CAD build for the part. Positions are in the model's coordinates, mm. A direction names the side the tool comes from. Coordinates: 2 decimals unless noted, no trailing zeros. Order: outer loops, then holes, each group sorted by start corner. A loop starts at its lowest first (then second) coordinate and runs counter-clockwise, first axis right, second up. Notation, with made-up numbers: (-23, -14.75) - (7, -14.75) arc R21 ccw to (7, -6.75) - close; hole circle Ø5 at (32, 23.5). An arc over 180 degrees is marked (long way). Use one line per item in the form item = value.
Autodesk Inventor part; units mm, degrees
ref_plane "YZ Plane" through (0, 0, 0) normal (1, 0, 0) x (0, 1, 0)
ref_plane "XZ Plane" through (0, 0, 0) normal (0, 1, 0) x (-1, 0, 0)
ref_plane "XY Plane" through (0, 0, 0) normal (0, 0, 1) x (1, 0, 0)
sketch "Sketch1" plane through (0, 0, 0) normal (0, 0, 1) x (1, 0, 0)
  line L0 (-5.7995, -0.4901) -> (0.2005, -0.4901)
  line L1 (0.2005, -0.4901) -> (0.2005, 2.5099)
  line L2 (0.2005, 2.5099) -> (10.2005, 2.5099)
  line L3 (10.2005, 2.5099) -> (10.2005, -0.4901)
  line L4 (10.2005, -0.4901) -> (16.2005, -0.4901)
  line L5 (16.2005, -0.4901) -> (16.2005, 1.5099)
  line L6 (16.2005, 1.5099) -> (12.2005, 1.5099)
  line L7 (12.2005, 1.5099) -> (12.2005, 4.5099)
  line L8 (12.2005, 4.5099) -> (-1.7995, 4.5099)
  line L9 (-1.7995, 4.5099) -> (-1.7995, 1.5099)
  line L10 (-1.7995, 1.5099) -> (-5.7995, 1.5099)
  line L11 (-5.7995, 1.5099) -> (-5.7995, -0.4901)
  point P0 (0, 0)
  dimension "d0" = 3
  dimension "d1" = 2
  dimension "d2" = 2
  dimension "d3" = 2
  dimension "d4" = 2
  dimension "d5" = 2
  dimension "d6" = 10
  dimension "d7" = 6
  dimension "d8" = 6
extrude "Extrusion1" add sketch "Sketch1" along normal blind 8
sketch "Sketch2" plane through (12.2005, 1.5099, 0) normal (0, 1, 0) x (1, 0, 0)
  line L0 (-14, 0) -> (-18, 0)
  line L1 (-18, 0) -> (-18, -8)
  line L2 (-14, -8) -> (-18, -8)
  line L3 (-14, 0) -> (-14, -8)
  line L4 (4, 0) -> (0, 0)
  line L5 (0, 0) -> (0, -8)
  line L6 (4, -8) -> (0, -8)
  line L7 (4, 0) -> (4, -8)
  point P0 (-12.2005, 0)
  point P1 (-16, -1.8)
  point P2 (-16, -6.2)
  point P3 (2, -1.8)
  point P4 (2, -6.2)
  dimension "d11" = 1.8
  dimension "d12" = 1.8
  dimension "d13" = 2
  dimension "d14" = 2
hole "Hole1" at (-3.7995, 1.5099, 1.8) at (-3.7995, 1.5099, 6.2) at (14.2005, 1.5099, 1.8) at (14.2005, 1.5099, 6.2) direction (0, -1, 0) diameter 1.6 depth 8 tip angle 118
fillet "Fillet1" radius 1.5 4 edges at (16.2005, 0.5099, 0) (16.2005, 0.5099, 8) (-5.7995, 0.5099, 0) (-5.7995, 0.5099, 8)
fillet "Fillet2" radius 0.25 4 edges at (12.2005, 4.5099, 4) (12.2005, 1.5099, 4) (-1.7995, 1.5099, 4) (-1.7995, 4.5099, 4)
chamfer "Chamfer1" distance 0.8 distance2 2 1 edges at (5.2005, 2.5099, 8) measured on face at (3.5338, 3.8432, 8)
chamfer "Chamfer2" distance 0.8 distance2 2 1 edges at (0.2005, 1.0099, 8) measured on face at (3.5338, 4.1099, 8)
chamfer "Chamfer3" distance 0.8 distance2 2 1 edges at (10.2005, 1.0099, 8) measured on face at (3.5338, 4.1099, 8)
equation "\"d2\" = d1"
equation "\"d3\" = d1"
equation "\"d4\" = d1"
equation "\"d5\" = d1"
equation "\"d7\" = d8"
properties part number "CNCM_ALU_Visial_inspection_tray_bucket_mount" material "Aluminum 6061"
Item 1: Cut at C-C, the plane x = -4. Write the cut outline in (y, z).
Derived:
outline = (-0.49, 0) - (1.51, 0) - (1.51, 1.03) - (-0.49, 1.03) - close; (-0.49, 2.57) - (1.51, 2.57) - (1.51, 5.43) - (-0.49, 5.43) - close; (-0.49, 6.97) - (1.51, 6.97) - (1.51, 8) - (-0.49, 8) - close
Item 2: Drop flat-ended pins along their axis: pin 1 (2 mm diameter, centred on y = 3, z = 7, fed in from -X); pin 2 (3 mm diameter, centred on x = 6.5, z = 4, fed in from -Y); pin 3 (0.8 mm diameter, centred on y = 3.5, z = 5.5, fed in from +X); pin 4 (1.4 mm diameter, centred on x = -3.8, z = 1.8, fed in from -Y). Give the stop position or say it passes through.
Derived:
pin_1 = -1.8
pin_2 = 2.51
pin_3 = 12.2
pin_4 = through
Item 3: Two-plate mould, pull along X, no slides. Class faces 1 (the face through (10.6, 1.4, 7)), 2 (the face through (-5.37, 0.5, 0.45)), 3 (the face through (5, 4.51, 4)): +X half, -X half, draft (parallel to the pull), parting line (faces both ways), or undercut.
Derived:
face_1 = undercut
face_2 = -X half
face_3 = draft
Item 4: Cut at D-D, the plane z = 4. Write the cut outline in (x, y).
Derived:
outline = (-5.8, -0.49) - (0.2, -0.49) - (0.2, 2.51) - (10.2, 2.51) - (10.2, -0.49) - (16.2, -0.49) - (16.2, 1.51) - (12.45, 1.51) arc R0.25 cw to (12.2, 1.76) - (12.2, 4.26) arc R0.25 ccw to (11.95, 4.51) - (-1.55, 4.51) arc R0.25 ccw to (-1.8, 4.26) - (-1.8, 1.76) arc R0.25 cw to (-2.05, 1.51) - (-5.8, 1.51) - close
Item 5: Drill centre lines: line 1 (X direction, y = 0.9, z = 1.8); line 2 (X direction, y = 0.3, z = 4.5); line 3 (X direction, y = 1, z = 6.2). Where is each one in solid material? Low to high. Write a range as [from, to].
Derived:
line_1 = [-5.8, -4.6], [-3, 0.2], [10.2, 13.4], [15, 16.2]
line_2 = [-5.8, 0.2], [10.2, 16.2]
line_3 = [-5.8, -4.6], [-3, 0.12], [10.28, 13.4], [15, 16.2]
Item 6: Cut at B-B, the plane y = 0.6. Write the cut outline in (x, z).
Derived:
outline = (-5.8, 1.5) arc R1.5 ccw to (-4.3, 0) - (0.2, 0) - (0.2, 6) - (-0.6, 8) - (-4.3, 8) arc R1.5 ccw to (-5.8, 6.5) - close; (10.2, 0) - (14.7, 0) arc R1.5 ccw to (16.2, 1.5) - (16.2, 6.5) arc R1.5 ccw to (14.7, 8) - (11, 8) - (10.2, 6) - close; hole circle Ø1.6 at (-3.8, 1.8); hole circle Ø1.6 at (-3.8, 6.2); hole circle Ø1.6 at (14.2, 1.8); hole circle Ø1.6 at (14.2, 6.2)
Item 7: Cut at A-A, the plane z = 1.8. Write the cut outline in (x, y), plus the area to 3 significant figures.
Derived:
outline = (-5.8, -0.49) - (-4.6, -0.49) - (-4.6, 1.51) - (-5.8, 1.51) - close; (-3, -0.49) - (0.2, -0.49) - (0.2, 2.51) - (10.2, 2.51) - (10.2, -0.49) - (13.4, -0.49) - (13.4, 1.51) - (12.45, 1.51) arc R0.25 cw to (12.2, 1.76) - (12.2, 4.26) arc R0.25 ccw to (11.95, 4.51) - (-1.55, 4.51) arc R0.25 ccw to (-1.8, 4.26) - (-1.8, 1.76) arc R0.25 cw to (-2.05, 1.51) - (-3, 1.51) - close; (15, -0.49) - (16.2, -0.49) - (16.2, 1.51) - (15, 1.51) - close
area = 49.6 mm²
Item 8: 3-axis set-ups, long thin cutter, end or side, ignore diameter. For faces 4 (the face through (-4, 1.51, 4)), 5 (the face through (5, 2.51, 3)), 6 (the face through (-0.2, 1.4, 7)): which of +Z, -Z, +X, -X, +Y, -Y reach the whole face in a straight line?
Derived:
face_4 = +Z, -Z, -X, +Y
face_5 = +Z, -Z, -Y
face_6 = +Z, -Y
